Verification items for the finished model (mm, model axes). A direction names the side the tool comes from. Round coordinates to 2 decimals unless told otherwise and drop trailing zeros. Order: outer loops, then holes, each group sorted by start corner. A loop starts at its lowest first (then second) coordinate and runs counter-clockwise, first axis right, second up. Notation, with made-up numbers: (56, 21) -> (84, 21) arc R29 ccw to (84, 42) -> close; hole circle Ø4 at (-23, -38.75). An arc over 180 degrees is marked (long way). Return JSON: item names as keys, results as strings. Group by question number.
1) Depth check by flat-ended pin: pin 1 (10 mm diameter, centred on x = -6.5, z = 5.5, fed in from +Y); pin 2 (8.5 mm diameter, centred on x = 0, y = 0, fed in from -Z); pin 3 (5 mm diameter, centred on y = -8, z = 13, fed in from -X). Enter the tip coordinate at first touch or a pass-through.
2) Draft check along X on faces 4 (the flat face through (-7, -2, 40)), 5 (the flat face through (0, -3, 35)), 6 (the cylindrical face through (-2.17, -9.76, 19.72)), 7 (the cylindrical face through (-6.466, -2.681, 2.465)). Enter one of: pulls with the +X half, pulls with the -X half, needs draft (parallel to the pull), parting line crosses it, or undercut.
3) Scan lines: L1, parallel to Y at x = 0, z = 27.25; L2, parallel to Z at x = -2.25, y = 3.5; L3, parallel to Y at x = 0, z = 1.4. Record each from-to range of solid material in increasing order.
4) Section check D-D on y = 5. Enter the section's corners in (x, z), plus the area to 3 significant figures.
5) Section check A-A on y = 0. Enter the section's corners in (x, z), plus the area to 3 significant figures.
6) Tool access check on faces 1 (the cylindrical face through (-6.466, -2.681, 37.535)), 2 (the flat face through (0, -3, 5)), 3 (the flat face through (-7, -2, 0)). Record the directions out of +Z, -Z, +X, -X, +Y, -Y that give a thin tool (end or side, any length) a straight path to the whole face; none if there is none.
7) Section check C-C on z = 27.5. Enter the section's corners in (x, y), plus the area to 3 significant figures.
```python
from build123d import *

# Parameters (mm, degrees)
SKETCH_1_R          = 10
SKETCH_1_R_2        = 2.5
EXTRUDE_1_DEPTH     = 40
SKETCH_2_R          = 7
CUT_EXTRUDE_1_DEPTH = 5


with BuildPart() as part:
    # 草图1 → 凸台-拉伸1 (new body)
    with BuildSketch(Plane.XY):
        Circle(SKETCH_1_R)
        Circle(SKETCH_1_R_2, mode=Mode.SUBTRACT)
    extrude(amount=EXTRUDE_1_DEPTH)

    # 草图2 → 切除-拉伸1 (cut)
    with BuildSketch(Plane(origin=(0, 0, 0), x_dir=(-1, 0, 0), z_dir=(0, 0, -1))):
        Circle(SKETCH_2_R)
    cut_extrude_1 = extrude(amount=-CUT_EXTRUDE_1_DEPTH, mode=Mode.SUBTRACT)

    # 镜向1: 切除-拉伸1 across plane
    add(cut_extrude_1.mirror(Plane.XY.offset(20)), mode=Mode.SUBTRACT)


solid = part.part
```
Check result:
{
 "1": {"pin 1": "y = 9.89", "pin 2": "z = 5", "pin 3": "x = -8.35"},
 "2": {"face 4": "needs draft", "face 5": "undercut", "face 6": "parting line crosses it", "face 7": "undercut"},
 "3": {"L1": "-10 to -2.5, 2.5 to 10", "L2": "5 to 35", "L3": "-10 to -7, 7 to 10"},
 "4": {"outline": "(-8.66, 0) -> (-4.9, 0) -> (-4.9, 5) -> (4.9, 5) -> (4.9, 0) -> (8.66, 0) -> (8.66, 40) -> (4.9, 40) -> (4.9, 35) -> (-4.9, 35) -> (-4.9, 40) -> (-8.66, 40) -> close", "area": "595 mm^2"},
 "5": {"outline": "(-10, 0) -> (-7, 0) -> (-7, 5) -> (-2.5, 5) -> (-2.5, 35) -> (-7, 35) -> (-7, 40) -> (-10, 40) -> close; (2.5, 5) -> (7, 5) -> (7, 0) -> (10, 0) -> (10, 40) -> (7, 40) -> (7, 35) -> (2.5, 35) -> close", "area": "510 mm^2"},
 "6": {"face 1": "+Z", "face 2": "-Z", "face 3": "-Z, +X, -X, +Y, -Y"},
 "7": {"outline": "circle Ø20 at (0, 0); hole circle Ø5 at (0, 0)", "area": "295 mm^2"}
}
